For this review, take the finished solid that the model builds, in its own axes (mm). Face numbers are marked on the shaded views. A direction names the side the tool comes from. Give positions to 0.01 mm unless a question says otherwise; leave off trailing zeros. Write each loop counter-clockwise with the first axis right and the second up, starting at its lowest first coordinate (ties: lowest second). Pieces come first, ordered by that corner, then holes. Notation, with made-up numbers: (-4.5, 53) -> (5.5, 53) arc R17 cw to (5.5, 65) -> close; hole circle Ø2 at (8, -38.5). An arc over 180 degrees is marked (long way). Write item = value, one per line.
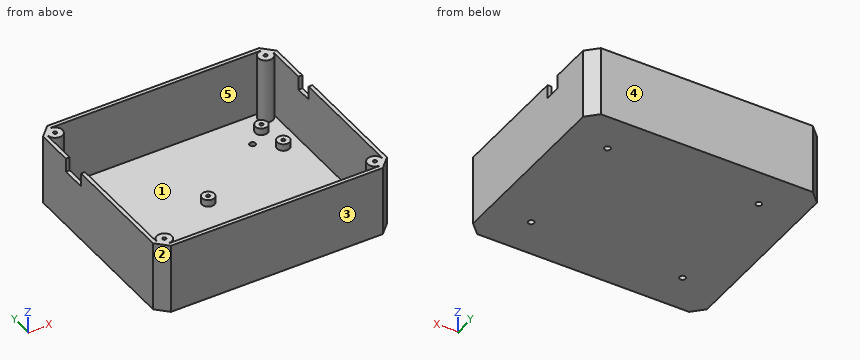
```python
from build123d import *

# Parameters (mm, degrees)
FLOOR_3_2_FOUR_CASE_MOUNTING_HOLES_2_R      = 2.15
FLOOR_3_2_FOUR_CASE_MOUNTING_HOLES_D4_DEPTH = 3.2
PERIMETER_START                             = 3.2
PERIMETER_WALL_2_8_DEPTH                    = 47.8
LID_START                                   = 3.2
LID_POST_CORES_PROFILE_R                    = 5.4
LID_POST_CORES_DEPTH                        = 37.8
LID_START_2                                 = 41
LID_POST_TIPS_D2_6_PILOT_X_10_PROFILE_R     = 5.4
LID_POST_TIPS_D2_6_PILOT_X_10_PROFILE_R_2   = 1.3
LID_POST_TIPS_D2_6_PILOT_X_10_DEPTH         = 10
TRAY_START                                  = 3.2
TRAY_SUPPORTS_D2_6_PILOT_X_5_PROFILE_R      = 4.5
TRAY_SUPPORTS_D2_6_PILOT_X_5_PROFILE_R_2    = 1.3
TRAY_SUPPORTS_D2_6_PILOT_X_5_DEPTH          = 5
CABLE_START                                 = 51
CABLE_EXITS_18_X_10_AND_12_X_10_PROFILE_W   = 6
CABLE_EXITS_18_X_10_AND_12_X_10_PROFILE_H   = 18
CABLE_EXITS_18_X_10_AND_12_X_10_PROFILE_H_2 = 12
CABLE_EXITS_18_X_10_AND_12_X_10_DEPTH       = 10


with BuildPart() as part:
    # Floor 3.2 - four case mounting holes 2 → Floor 3.2 - four case mounting holes D4 (new body)
    with BuildSketch(Plane.XY):
        Polygon((-77, -73), (77, -73), (85, -65), (85, 65), (77, 73), (-77, 73), (-85, 65), (-85, -65), align=None)
        with Locations((-55, -45)):
            Circle(FLOOR_3_2_FOUR_CASE_MOUNTING_HOLES_2_R, mode=Mode.SUBTRACT)
        with Locations((-55, 45)):
            Circle(FLOOR_3_2_FOUR_CASE_MOUNTING_HOLES_2_R, mode=Mode.SUBTRACT)
        with Locations((55, -45)):
            Circle(FLOOR_3_2_FOUR_CASE_MOUNTING_HOLES_2_R, mode=Mode.SUBTRACT)
        with Locations((55, 45)):
            Circle(FLOOR_3_2_FOUR_CASE_MOUNTING_HOLES_2_R, mode=Mode.SUBTRACT)
    extrude(amount=FLOOR_3_2_FOUR_CASE_MOUNTING_HOLES_D4_DEPTH)

    # Perimeter wall 2.8 profile → Perimeter wall 2.8 (add)
    with BuildSketch(Plane.XY.offset(PERIMETER_START)):
        Polygon((-77, -73), (77, -73), (85, -65), (85, 65), (77, 73), (-77, 73), (-85, 65), (-85, -65), align=None)
        Polygon((-75.84, -70.2), (75.84, -70.2), (82.2, -63.84), (82.2, 63.84), (75.84, 70.2), (-75.84, 70.2), (-82.2, 63.84), (-82.2, -63.84), align=None, mode=Mode.SUBTRACT)
    extrude(amount=PERIMETER_WALL_2_8_DEPTH)

    # Lid post cores profile → Lid post cores (add)
    with BuildSketch(Plane.XY.offset(LID_START)):
        with Locations((-76.5, -64.5)):
            Circle(LID_POST_CORES_PROFILE_R)
        with Locations((-76.5, 64.5)):
            Circle(LID_POST_CORES_PROFILE_R)
        with Locations((76.5, -64.5)):
            Circle(LID_POST_CORES_PROFILE_R)
        with Locations((76.5, 64.5)):
            Circle(LID_POST_CORES_PROFILE_R)
    extrude(amount=LID_POST_CORES_DEPTH)

    # Lid post tips - D2.6 pilot x 10 profile → Lid post tips - D2.6 pilot x 10 (add)
    # profile 1 of 4: a face of its own
    with BuildSketch(Plane.XY.offset(LID_START_2)):
        with Locations((-76.5, -64.5)):
            Circle(LID_POST_TIPS_D2_6_PILOT_X_10_PROFILE_R)
        with Locations((-76.5, -64.5)):
            Circle(LID_POST_TIPS_D2_6_PILOT_X_10_PROFILE_R_2, mode=Mode.SUBTRACT)
    # profile 2 of 4: a face of its own
    with BuildSketch(Plane.XY.offset(LID_START_2)):
        with Locations((-76.5, 64.5)):
            Circle(LID_POST_TIPS_D2_6_PILOT_X_10_PROFILE_R)
        with Locations((-76.5, 64.5)):
            Circle(LID_POST_TIPS_D2_6_PILOT_X_10_PROFILE_R_2, mode=Mode.SUBTRACT)
    # profile 3 of 4: a face of its own
    with BuildSketch(Plane.XY.offset(LID_START_2)):
        with Locations((76.5, -64.5)):
            Circle(LID_POST_TIPS_D2_6_PILOT_X_10_PROFILE_R)
        with Locations((76.5, -64.5)):
            Circle(LID_POST_TIPS_D2_6_PILOT_X_10_PROFILE_R_2, mode=Mode.SUBTRACT)
    # profile 4 of 4: a face of its own
    with BuildSketch(Plane.XY.offset(LID_START_2)):
        with Locations((76.5, 64.5)):
            Circle(LID_POST_TIPS_D2_6_PILOT_X_10_PROFILE_R)
        with Locations((76.5, 64.5)):
            Circle(LID_POST_TIPS_D2_6_PILOT_X_10_PROFILE_R_2, mode=Mode.SUBTRACT)
    extrude(amount=LID_POST_TIPS_D2_6_PILOT_X_10_DEPTH)

    # Tray supports - D2.6 pilot x 5 profile → Tray supports - D2.6 pilot x 5 (add)
    # profile 1 of 6: a face of its own
    with BuildSketch(Plane.XY.offset(TRAY_START)):
        with Locations((-67, -55)):
            Circle(TRAY_SUPPORTS_D2_6_PILOT_X_5_PROFILE_R)
        with Locations((-67, -55)):
            Circle(TRAY_SUPPORTS_D2_6_PILOT_X_5_PROFILE_R_2, mode=Mode.SUBTRACT)
    # profile 2 of 6: a face of its own
    with BuildSketch(Plane.XY.offset(TRAY_START)):
        with Locations((-67, 54)):
            Circle(TRAY_SUPPORTS_D2_6_PILOT_X_5_PROFILE_R)
        with Locations((-67, 54)):
            Circle(TRAY_SUPPORTS_D2_6_PILOT_X_5_PROFILE_R_2, mode=Mode.SUBTRACT)
    # profile 3 of 6: a face of its own
    with BuildSketch(Plane.XY.offset(TRAY_START)):
        with Locations((67, -55)):
            Circle(TRAY_SUPPORTS_D2_6_PILOT_X_5_PROFILE_R)
        with Locations((67, -55)):
            Circle(TRAY_SUPPORTS_D2_6_PILOT_X_5_PROFILE_R_2, mode=Mode.SUBTRACT)
    # profile 4 of 6: a face of its own
    with BuildSketch(Plane.XY.offset(TRAY_START)):
        with Locations((67, 54)):
            Circle(TRAY_SUPPORTS_D2_6_PILOT_X_5_PROFILE_R)
        with Locations((67, 54)):
            Circle(TRAY_SUPPORTS_D2_6_PILOT_X_5_PROFILE_R_2, mode=Mode.SUBTRACT)
    # profile 5 of 6: a face of its own
    with BuildSketch(Plane.XY.offset(TRAY_START)):
        with Locations((0, 8)):
            Circle(TRAY_SUPPORTS_D2_6_PILOT_X_5_PROFILE_R)
        with Locations((0, 8)):
            Circle(TRAY_SUPPORTS_D2_6_PILOT_X_5_PROFILE_R_2, mode=Mode.SUBTRACT)
    # profile 6 of 6: a face of its own
    with BuildSketch(Plane.XY.offset(TRAY_START)):
        with Locations((70, 33)):
            Circle(TRAY_SUPPORTS_D2_6_PILOT_X_5_PROFILE_R)
        with Locations((70, 33)):
            Circle(TRAY_SUPPORTS_D2_6_PILOT_X_5_PROFILE_R_2, mode=Mode.SUBTRACT)
    extrude(amount=TRAY_SUPPORTS_D2_6_PILOT_X_5_DEPTH)

    # Cable exits 18 x 10 and 12 x 10 profile → Cable exits 18 x 10 and 12 x 10 (cut)
    with BuildSketch(Plane.XY.offset(CABLE_START)):
        with Locations((-84, 29)):
            Rectangle(CABLE_EXITS_18_X_10_AND_12_X_10_PROFILE_W, CABLE_EXITS_18_X_10_AND_12_X_10_PROFILE_H)
        with Locations((84, 29)):
            Rectangle(CABLE_EXITS_18_X_10_AND_12_X_10_PROFILE_W, CABLE_EXITS_18_X_10_AND_12_X_10_PROFILE_H_2)
    extrude(amount=-CABLE_EXITS_18_X_10_AND_12_X_10_DEPTH, mode=Mode.SUBTRACT)


solid = part.part
```
(1) Tool access review of the marked faces 1 and 2: name each direction out of +Z, -Z, +X, -X, +Y, -Y from which nothing blocks a thin tool from reaching the whole face with its end or side.
Answers below:
face_1 = +Z
face_2 = +Z, -Z, -X, -Y
(2) To check wall thickness, follow probe 1 along Y at (x, z) = (-67, 6); probe 2 along Y at (x, z) = (55, 1.8); probe 3 along Y at (x, z) = (76, 18). State the ranges of each line that lie inside material, in increasing order.
Answers below:
probe_1 = -73 to -70.2, -59.5 to -56.3, -53.7 to -50.5, 49.5 to 52.7, 55.3 to 58.5, 70.2 to 73
probe_2 = -73 to -47.15, -42.85 to 42.85, 47.15 to 73
probe_3 = -73 to -70.04, -69.88 to -59.12, 59.12 to 69.88, 70.04 to 73
(3) Take a section at A-A (z = 22.5). Write out the cut boundary in (x, y).
Answers below:
outline = (-85, -65) -> (-77, -73) -> (77, -73) -> (85, -65) -> (85, 65) -> (77, 73) -> (-77, 73) -> (-85, 65) -> close; hole (-82.2, -63.84) -> (-81.89, -64.15) arc R5.4 cw (long way) to (-76.15, -69.89) -> (-75.84, -70.2) -> (75.84, -70.2) -> (76.15, -69.89) arc R5.4 cw (long way) to (81.89, -64.15) -> (82.2, -63.84) -> (82.2, 63.84) -> (81.89, 64.15) arc R5.4 cw (long way) to (76.15, 69.89) -> (75.84, 70.2) -> (-75.84, 70.2) -> (-76.15, 69.89) arc R5.4 cw (long way) to (-81.89, 64.15) -> (-82.2, 63.84) -> close
(4) The part is to be moulded in two halves that separate along Y. For the marked faces 3, 4 and 5, say which applies: released by +Y, released by -Y, zero draft, split by the parting line, or undercut.
Answers below:
face_3 = released by -Y
face_4 = released by +Y
face_5 = undercut
(5) Take a section at D-D (y = 1). Write out the cut boundary in (x, z).
Answers below:
outline = (-85, 0) -> (85, 0) -> (85, 51) -> (82.2, 51) -> (82.2, 3.2) -> (-82.2, 3.2) -> (-82.2, 51) -> (-85, 51) -> close
(6) Take a section at C-C (x = 55). Write out the cut boundary in (y, z), plus the area to 3 significant figures.
Answers below:
outline = (-73, 0) -> (-47.15, 0) -> (-47.15, 3.2) -> (-70.2, 3.2) -> (-70.2, 51) -> (-73, 51) -> close; (-42.85, 0) -> (42.85, 0) -> (42.85, 3.2) -> (-42.85, 3.2) -> close; (47.15, 0) -> (73, 0) -> (73, 51) -> (70.2, 51) -> (70.2, 3.2) -> (47.15, 3.2) -> close
area = 707 mm^2
(7) Take a section at B-B (y = 45). Write out the cut boundary in (x, z), plus the area to 3 significant figures.
Answers below:
outline = (-85, 0) -> (-57.15, 0) -> (-57.15, 3.2) -> (-82.2, 3.2) -> (-82.2, 51) -> (-85, 51) -> close; (-52.85, 0) -> (52.85, 0) -> (52.85, 3.2) -> (-52.85, 3.2) -> close; (57.15, 0) -> (85, 0) -> (85, 51) -> (82.2, 51) -> (82.2, 3.2) -> (57.15, 3.2) -> close
area = 784 mm^2
(8) For pin 1 (0.8 mm diameter, centred on x = 70, y = 33, fed in from +Z); pin 2 (10 mm diameter, centred on x = 71, y = 35, fed in from +Z); pin 3 (3 mm diameter, centred on x = -84, z = 44.5, fed in from -Y); pin 4 (2.5 mm diameter, centred on x = 55, y = 45, fed in from +Z), all flat-tipped, find the tip position at first contact; note any pin that passes through.
Answers below:
pin_1 = 3.2
pin_2 = 8.2
pin_3 = -67.5
pin_4 = through
